Could you check a few things on this model? Use its own coordinates, in mm. A direction names the side the tool comes from. Coordinates: 2 decimals unless noted, no trailing zeros. Loops run counter-clockwise (first coordinate to the right, second up) from the corner with the lowest first, then second, coordinate; pieces in that order, holes last.
1) Imagine slicing it at A-A on y = 6. Please give me the cut outline in (x, z).
2) Imagine slicing it at D-D on z = -33.5. Please give me the cut outline in (x, y).
3) Imagine slicing it at C-C on z = -39. Please give me the cut outline in (x, y).
4) Thinking about a two-plate mould opening in Y: for faces 6 (the face through (-5, 1, -11)), 7 (the face through (-1, 3, -40)), 8 (the face through (-5, 9, -11)), 9 (the face through (-0.466, 5.056, -2.709)), which applies, released by +Y, released by -Y, zero draft, split by the parting line, or undercut?
5) For faces 1 (the face through (-48.447, 7.986, -2.317)), 2 (the face through (-1, 7, -40)), 3 (the face through (-28, 5, -8.449)), 4 (the face through (-2.361, 2.014, -44.447)), 5 (the face through (-40, 7, -3)), which set-ups out of +Z, -Z, +X, -X, +Y, -Y let a thin tool reach every point of the face, with its end or its side?
6) Imagine slicing it at B-B on x = -38. Please give me the cut outline in (y, z).
7) Will these pins go through, and if not, where does the flat tip stop? P1, Ø3, axis at x = -3.5, y = 4, coming from the -Z side; P2, Ø4.5, axis at y = 4.5, z = -5, coming from the -X side; P3, Ø4, axis at y = 6.5, z = -32, coming from the -X side.
8) If I drill on line 1 along Y through (x, z) = (-5.5, -37); line 2 along X through (y, z) = (6, -16.5); line 3 along Z through (x, y) = (-43, 1.75), over which ranges is the centre line in solid material (lowest first)?
```python
from build123d import *

# Parameters (mm, degrees)
SKETCH1_R               = 2.4
BOSS_EXTRUDE1_DEPTH     = 10
CUT_EXTRUDE1_DEPTH      = 2.5
CUT_EXTRUDE1_DEPTH_BACK = 2.5
SKETCH2_R               = 2.4
CUT_EXTRUDE2_DEPTH      = 2.5
CUT_EXTRUDE2_DEPTH_BACK = 2.5
SKETCH3_R               = 2.4
SCALE1_SCALE            = 0.8
SKETCH4_R               = 2
CUT_EXTRUDE3_DEPTH      = 69.982589006


with BuildPart() as part:
    # Sketch1 → Boss-Extrude1 (new body)
    with BuildSketch(Plane(origin=(0, 0, 0), x_dir=(1, 0, 0), z_dir=(0, 1, 0))):
        with BuildLine():
            Line((-50, 7.5), (-12.5, 7.5))
            ThreePointArc((-12.5, 7.5), (-8.964466094, 8.964466094), (-7.5, 12.5))
            Line((-7.5, 12.5), (-7.5, 50))
            ThreePointArc((-7.5, 50), (0, 57.5), (7.5, 50))
            Line((7.5, 50), (7.5, 0))
            ThreePointArc((7.5, 0), (5.303300859, -5.303300859), (0, -7.5))
            Line((0, -7.5), (-50, -7.5))
            ThreePointArc((-50, -7.5), (-57.5, 0), (-50, 7.5))
        make_face()
        with Locations(Location((0, 0, 0), (0, 0, 270))):
            Circle(SKETCH1_R, mode=Mode.SUBTRACT)
        with Locations(Location((-50, 0, 0), (0, 0, 270))):
            Circle(SKETCH1_R, mode=Mode.SUBTRACT)
        with Locations(Location((0, 50, 0), (0, 0, 270))):
            Circle(SKETCH1_R, mode=Mode.SUBTRACT)
    extrude(amount=BOSS_EXTRUDE1_DEPTH)

    # Sketch2 → Cut-Extrude1 (cut, two sides: drawn at the far end of the back side and taken through both)
    with BuildSketch(Plane(origin=(0, 5, 0), x_dir=(1, 0, 0), z_dir=(0, 1, 0)).offset(-CUT_EXTRUDE1_DEPTH_BACK)):
        with BuildLine():
            Line((-50, 7.5), (-41, 7.5))
            Line((-41, 7.5), (-41, -7.5))
            Line((-41, -7.5), (-50, -7.5))
            ThreePointArc((-50, -7.5), (-57.5, 0), (-50, 7.5))
        make_face()
        with Locations(Location((-50, 0, 0), (0, 0, 270))):
            Circle(SKETCH2_R, mode=Mode.SUBTRACT)
    extrude(amount=CUT_EXTRUDE1_DEPTH + CUT_EXTRUDE1_DEPTH_BACK, mode=Mode.SUBTRACT)

    # Sketch3 → Cut-Extrude2 (cut, two sides: drawn at the far end of the back side and taken through both)
    with BuildSketch(Plane(origin=(0, 5, 0), x_dir=(1, 0, 0), z_dir=(0, 1, 0)).offset(-CUT_EXTRUDE2_DEPTH_BACK)):
        with BuildLine():
            Line((-7.5, 50), (-7.5, 41))
            Line((-7.5, 41), (7.5, 41))
            Line((7.5, 41), (7.5, 50))
            ThreePointArc((7.5, 50), (0, 57.5), (-7.5, 50))
        make_face()
        with Locations(Location((0, 50, 0), (0, 0, 270))):
            Circle(SKETCH3_R, mode=Mode.SUBTRACT)
    extrude(amount=CUT_EXTRUDE2_DEPTH + CUT_EXTRUDE2_DEPTH_BACK, mode=Mode.SUBTRACT)


with BuildPart() as part_1:
    # Scale1: scaled about (-12.244648703, 5, -12.244648703)
    add(part.part.scale(SCALE1_SCALE).moved(Location((-2.448929741, 1, -2.448929741))))

    # Sketch4 → Cut-Extrude3 (cut, through all)
    with BuildSketch(Plane(origin=(0, 9, 0), x_dir=(1, 0, 0), z_dir=(0, 1, 0))):
        with Locations(Location((-2.448929741, 42.448929741, 0), (0, 0, 270))):
            Circle(SKETCH4_R)
        with Locations(Location((-2.448929741, 2.448929741, 0), (0, 0, 270))):
            Circle(SKETCH4_R)
        with Locations(Location((-42.448929741, 2.448929741, 0), (0, 0, 270))):
            Circle(SKETCH4_R)
    extrude(amount=-CUT_EXTRUDE3_DEPTH, mode=Mode.SUBTRACT)


solid = part_1.part
```
Filled in:
1. outline: (-35.25, -8.45) - (-12.45, -8.45) arc R4 cw to (-8.45, -12.45) - (-8.45, -35.25) - (3.55, -35.25) - (3.55, -2.45) arc R6 ccw to (-2.45, 3.55) - (-35.25, 3.55) - close; hole circle Ø4 at (-2.45, -2.45)
2. outline: (-8.45, 1) - (3.55, 1) - (3.55, 9) - (-8.45, 9) - close
3. outline: (-8.45, 1) - (3.55, 1) - (3.55, 3) - (-8.45, 3) - close; (-8.45, 7) - (3.55, 7) - (3.55, 9) - (-8.45, 9) - close
4. face 6: released by -Y
4. face 7: undercut
4. face 8: released by +Y
4. face 9: zero draft
5. face 1: -X, +Y, -Y
5. face 2: -Z, +X, -X
5. face 3: -Z, -X, +Y, -Y
5. face 4: +Y, -Y
5. face 5: +Z, -Z, -X
6. outline: (1, -8.45) - (3, -8.45) - (3, 3.55) - (1, 3.55) - close; (7, -8.45) - (9, -8.45) - (9, 3.55) - (7, 3.55) - close
7. P1: stops at z = -48.45
7. P2: stops at x = -48.38
7. P3: stops at x = -8.45
8. line 1: y = 1 to 3, 7 to 9
8. line 2: x = -8.45 to 3.55
8. line 3: z = -8.42 to -4.37, -0.53 to 3.53
